```python
from build123d import *

# Parameters (mm, degrees)
BOSS_EXTRUDE1_DEPTH      = 20
BOSS_EXTRUDE1_DEPTH_BACK = 20
SKETCH7_R                = 5.5
CUT_EXTRUDE5_DEPTH       = 20
FILLET8_R                = 20


with BuildPart() as part:
    # Sketch1 → Boss-Extrude1 (new, two sides: drawn at the far end of the back side and taken through both)
    with BuildSketch(Plane.XY.offset(-BOSS_EXTRUDE1_DEPTH_BACK)):
        with BuildLine():
            Line((35, 0), (74, 0))
            Line((74, 0), (74, 20))
            Line((74, 20), (42, 20))
            Line((42, 20), (42, 23.237900077))
            ThreePointArc((42, 23.237900077), (0, 48), (-42, 23.237900077))
            Line((-42, 23.237900077), (-42, 20))
            Line((-42, 20), (-74, 20))
            Line((-74, 20), (-74, 0))
            Line((-74, 0), (-35, 0))
            ThreePointArc((-35, 0), (0, 35), (35, 0))
        make_face()
    extrude(amount=BOSS_EXTRUDE1_DEPTH + BOSS_EXTRUDE1_DEPTH_BACK)

    # Sketch7 → Cut-Extrude5 (cut)
    with BuildSketch(Plane(origin=(0, 20, 0), x_dir=(1, 0, 0), z_dir=(0, 1, 0))):
        with Locations(Location((54, 0, 0), (0, 0, 270))):
            Circle(SKETCH7_R)
        with Locations(Location((-54, 0, 0), (0, 0, 270))):
            Circle(SKETCH7_R)
    extrude(amount=-CUT_EXTRUDE5_DEPTH, mode=Mode.SUBTRACT)

    # Fillet8
    fillet8_edges = [part.edges().sort_by_distance(p)[0] for p in [
        (-74, 10, -20),
        (-74, 10, 20),
        (74, 10, -20),
        (74, 10, 20),
    ]]
    fillet(fillet8_edges, radius=FILLET8_R - 0.0001)  # a hair under: the kernel refuses the full size


solid = part.part
```
Can you work these out from the model? Positions are in its coordinate system, mm. A direction names the side the tool comes from. Coordinates: 2 decimals unless noted, no trailing zeros. Loops run counter-clockwise (first coordinate to the right, second up) from the corner with the lowest first, then second, coordinate; pieces in that order, holes last. Notation, with made-up numbers: (31.25, -26) - (85.25, -26) arc R35 ccw to (85.25, 11) - close; hole circle Ø1 at (-33.5, -9.5). An arc over 180 degrees is marked (long way). Use a Markdown table: item, result.
Item 1: We'd pull the mould along X, two halves only. Please class faces 1 (the face through (67.986, 10.14, -14.297)), 2 (the face through (-0.77, 34.99, -0.28)), 3 (the face through (-67.986, 9.86, 14.297)), 4 (the face through (50, 0, 4)): released by +X, released by -X, zero draft, split by the parting line, or undercut.
Numbers:
| item | result |
|---|---|
| face 1 | released by +X |
| face 2 | undercut |
| face 3 | released by -X |
| face 4 | zero draft |
Item 2: I want a section at C-C on y = 27.5. Please give me the cut outline in (x, z).
Numbers:
| item | result |
|---|---|
| outline | (-39.34, -20) - (-21.65, -20) - (-21.65, 20) - (-39.34, 20) - close; (21.65, -20) - (39.34, -20) - (39.34, 20) - (21.65, 20) - close |
Item 3: I want a section at A-A on y = 6. Give the number of separate pieces and of enclosed holes in the cut face, and give its area (3 significant figures).
Numbers:
| item | result |
|---|---|
| separate pieces | 2 |
| enclosed holes | 2 |
| area | 2,630 mm2 |
Item 4: I want a section at B-B on z = -1.5. Please give me the cut outline in (x, y).
Numbers:
| item | result |
|---|---|
| outline | (-73.94, 0) - (-59.29, 0) - (-59.29, 20) - (-73.94, 20) - close; (-48.71, 0) - (-35, 0) arc R35 cw to (35, 0) - (48.71, 0) - (48.71, 20) - (42, 20) - (42, 23.24) arc R48 ccw to (-42, 23.24) - (-42, 20) - (-48.71, 20) - close; (59.29, 0) - (73.94, 0) - (73.94, 20) - (59.29, 20) - close |
Item 5: For faces 5 (the face through (59.453, 10.14, -0.716)), 6 (the face through (-42, 22, 0)), 7 (the face through (58, 20, 4)), which set-ups out of +Z, -Z, +X, -X, +Y, -Y let a thin tool reach every point of the face, with its end or its side?
Numbers:
| item | result |
|---|---|
| face 5 | +Y, -Y |
| face 6 | +Z, -Z, -X, +Y |
| face 7 | +Z, -Z, +X, +Y |
Item 6: If I drill on probe 1 along X at (y, z) = (15.75, 0); probe 2 along X at (y, z) = (7, 1); probe 3 along X at (y, z) = (13.5, -15), over which ranges is the centre line in solid material (lowest first)? Write a range as from..to.
Numbers:
| item | result |
|---|---|
| probe 1 | x = -74..-59.5, -48.5..-31.26, 31.26..48.5, 59.5..74 |
| probe 2 | x = -73.97..-59.41, -48.59..-34.29, 34.29..48.59, 59.41..73.97 |
| probe 3 | x = -67.23..-32.29, 32.29..67.23 |
Item 7: I want a section at D-D on z = -12. Please give me the cut outline in (x, y), and give its area (3 significant figures).
Numbers:
| item | result |
|---|---|
| outline | (-70, 0) - (-35, 0) arc R35 cw to (35, 0) - (70, 0) - (70, 20) - (42, 20) - (42, 23.24) arc R48 ccw to (-42, 23.24) - (-42, 20) - (-70, 20) - close |
| area | 2,630 mm2 |
Item 8: Will these pins go through, and if not, where does the flat tip stop? pin 1 (9.5 mm diameter, centred on x = -53, z = -5.5, fed in from +Y); pin 2 (2.5 mm diameter, centred on y = 22, z = -4, fed in from -X); pin 3 (4 mm diameter, centred on x = -17, z = 3, fed in from -Y).
Numbers:
| item | result |
|---|---|
| pin 1 | stops at y = 20 |
| pin 2 | stops at x = -42 |
| pin 3 | stops at y = 29.39 |
